Part model, mm, in its own coordinate system. Face numbers are marked on the shaded views. A direction names the side the tool comes from. Give positions to 0.01 mm unless a question says otherwise; leave off trailing zeros. Order: outer loops, then holes, each group sorted by start corner. A loop starts at its lowest first (then second) coordinate and runs counter-clockwise, first axis right, second up.
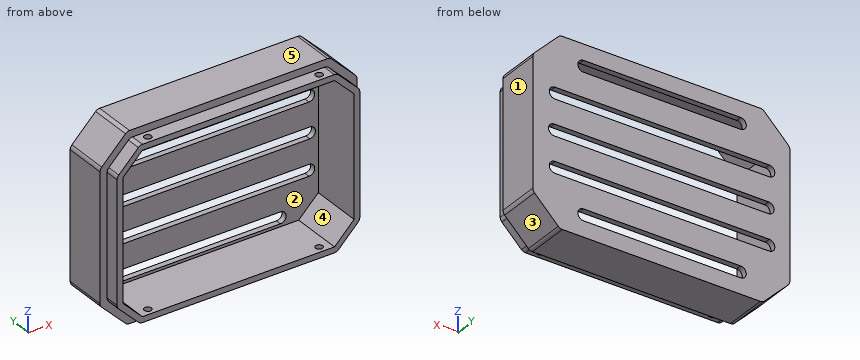
from build123d import *

# Parameters (mm, degrees)
BOSS_EXTRUDE1_DEPTH = 25.4
CUT_EXTRUDE1_DEPTH  = 6.35
CUT_EXTRUDE2_DEPTH  = 22.86
SKETCH4_R           = 1.575
CUT_EXTRUDE3_DEPTH  = 102.052823439
CUT_EXTRUDE4_DEPTH  = 75.93269063
FILLET1_R           = 2.54


with BuildPart() as part:
    # Sketch1 → Boss-Extrude1 (new body)
    with BuildSketch(Plane(origin=(0, 0, 0), x_dir=(1, 0, 0), z_dir=(0, 1, 0))):
        Polygon((-45.085, -41.275), (-57.15, -29.21), (-57.15, 29.21), (-45.085, 41.275), (45.085, 41.275), (57.15, 29.21), (57.15, -29.21), (45.085, -41.275), align=None)
    extrude(amount=BOSS_EXTRUDE1_DEPTH)

    # Sketch2 → Cut-Extrude1 (cut)
    with BuildSketch(Plane.XZ):
        Polygon((-57.15, 29.21), (-57.15, -29.21), (-45.085, -41.275), (45.085, -41.275), (57.15, -29.21), (57.15, 29.21), (45.085, 41.275), (-45.085, 41.275), align=None)
        Polygon((-53.975, 27.894871939), (-53.975, -27.894871939), (-43.769871939, -38.1), (43.769871939, -38.1), (53.975, -27.894871939), (53.975, 27.894871939), (43.769871939, 38.1), (-43.769871939, 38.1), align=None, mode=Mode.SUBTRACT)
    extrude(amount=-CUT_EXTRUDE1_DEPTH, mode=Mode.SUBTRACT)

    # Sketch3 → Cut-Extrude2 (cut)
    with BuildSketch(Plane.XZ):
        Polygon((-51.435, 26.842769491), (-51.435, -26.842769491), (-42.717769491, -35.56), (42.717769491, -35.56), (51.435, -26.842769491), (51.435, 26.842769491), (42.717769491, 35.56), (-42.717769491, 35.56), align=None)
    extrude(amount=-CUT_EXTRUDE2_DEPTH, mode=Mode.SUBTRACT)

    # Sketch4 → Cut-Extrude3 (cut, through all)
    with BuildSketch(Plane.XY.offset(38.1)):
        with Locations((-38.1, 3.175)):
            Circle(SKETCH4_R)
        with Locations((38.1, 3.175)):
            Circle(SKETCH4_R)
    extrude(amount=-CUT_EXTRUDE3_DEPTH, mode=Mode.SUBTRACT)

    # Sketch5 → Cut-Extrude4 (cut, through all)
    with BuildSketch(Plane(origin=(0, 25.4, 0), x_dir=(1, 0, 0), z_dir=(0, 1, 0))):
        with BuildLine():
            Line((-35.239850105, 34.29), (34.610149895, 34.29))
            ThreePointArc((34.610149895, 34.29), (37.150149895, 31.75), (34.610149895, 29.21))
            Line((34.610149895, 29.21), (-35.239850105, 29.21))
            ThreePointArc((-35.239850105, 29.21), (-37.779850105, 31.75), (-35.239850105, 34.29))
        make_face()
        with BuildLine():
            Line((-47.625, 2.54), (47.625, 2.54))
            ThreePointArc((47.625, 2.54), (50.165, 0), (47.625, -2.54))
            Line((47.625, -2.54), (-47.625, -2.54))
            ThreePointArc((-47.625, -2.54), (-50.165, 0), (-47.625, 2.54))
        make_face()
        with BuildLine():
            Line((-35.239850105, -29.21), (34.610149895, -29.21))
            ThreePointArc((34.610149895, -29.21), (37.150149895, -31.75), (34.610149895, -34.29))
            Line((34.610149895, -34.29), (-35.239850105, -34.29))
            ThreePointArc((-35.239850105, -34.29), (-37.779850105, -31.75), (-35.239850105, -29.21))
        make_face()
        with BuildLine():
            Line((-47.939850105, -13.335), (47.310149895, -13.335))
            ThreePointArc((47.310149895, -13.335), (49.850149895, -15.875), (47.310149895, -18.415))
            Line((47.310149895, -18.415), (-47.939850105, -18.415))
            ThreePointArc((-47.939850105, -18.415), (-50.479850105, -15.875), (-47.939850105, -13.335))
        make_face()
        with BuildLine():
            Line((-47.939850105, 18.415), (47.310149895, 18.415))
            ThreePointArc((47.310149895, 18.415), (49.850149895, 15.875), (47.310149895, 13.335))
            Line((47.310149895, 13.335), (-47.939850105, 13.335))
            ThreePointArc((-47.939850105, 13.335), (-50.479850105, 15.875), (-47.939850105, 18.415))
        make_face()
    extrude(amount=-CUT_EXTRUDE4_DEPTH, mode=Mode.SUBTRACT)

    # Fillet1
    fillet1_edges = [part.edges().sort_by_distance(p)[0] for p in [
        (-45.085, 15.875, 41.275),
        (-57.15, 15.875, 29.21),
        (-57.15, 15.875, -29.21),
        (-45.085, 15.875, -41.275),
        (45.085, 15.875, -41.275),
        (57.15, 15.875, -29.21),
        (57.15, 15.875, 29.21),
        (45.085, 15.875, 41.275),
        (-43.769871939, 3.175, 38.1),
        (43.769871939, 3.175, 38.1),
        (53.975, 3.175, 27.894871939),
        (53.975, 3.175, -27.894871939),
        (43.769871939, 3.175, -38.1),
        (-43.769871939, 3.175, -38.1),
        (-53.975, 3.175, -27.894871939),
        (-53.975, 3.175, 27.894871939),
    ]]
    fillet(fillet1_edges, radius=FILLET1_R)


solid = part.part
Item 1: Band-saw the part on A-A on x = 16. Give the number of separate pieces and of enclosed holes in the cut face, plus the area to 3 significant figures.
Item 2: Pull direction X, two halves, no side cores. Call the marked faces 3, 4 and 5: released by +X, released by -X, zero draft, split by the parting line, or undercut.
Item 3: Drill centre lines: probe 1 along X at (y, z) = (15.75, 20) (3 decimals); probe 2 along Z at (x, y) = (33.5, 23.5) (3 decimals); probe 3 along Z at (x, y) = (35, 4.25). Where is each one in solid material? Low to high.
Item 4: Band-saw the part on B-B on z = 0. List the corners of the cut face in (x, y) (3 decimals), plus the area to 3 significant figures.
Item 5: Drop flat-ended pins along their axis: P1, Ø8, axis at x = -4, z = -30.5, coming from the -Y side; P2, Ø3, axis at x = 12.5, y = 4, coming from the +Z side; P3, Ø3, axis at x = -3.5, y = 4, coming from the -Z side; P4, Ø5, axis at y = 4.5, z = 6, coming from the -X side. Give the stop position or say it passes through.
Item 6: Which spindle directions (+Z, -Z, +X, -X, +Y, -Y) get a long thin tool onto all of the face, cutting with end or side? Do the marked faces 1 and 2. Say none if no direction does.
Item 7: Band-saw the part on C-C on y = 19.75. List the corners of the cut face in (x, z) (3 decimals).
Item 8: Band-saw the part on D-D on z = 8.5. List the corners of the cut face in (x, y) (3 decimals), plus the area to 3 significant figures.
Working result:
1. separate pieces: 6
1. enclosed holes: 0
1. area: 366 mm2
2. face 3: released by +X
2. face 4: undercut
2. face 5: zero draft
3. probe 1: x = -57.15 to -51.435, 51.435 to 57.15
3. probe 2: z = -41.275 to -34.29, -29.21 to -18.415, -13.335 to -2.54, 2.54 to 13.335, 18.415 to 29.21, 34.29 to 41.275
3. probe 3: z = -38.1 to -35.56, 35.56 to 38.1
4. outline: (-57.15, 6.35) - (-53.975, 6.35) - (-53.975, 0) - (-51.435, 0) - (-51.435, 22.86) - (-50.165, 22.86) - (-50.165, 25.4) - (-57.15, 25.4) - close; (50.165, 22.86) - (51.435, 22.86) - (51.435, 0) - (53.975, 0) - (53.975, 6.35) - (57.15, 6.35) - (57.15, 25.4) - (50.165, 25.4) - close
4. area: 256 mm2
5. P1: stops at y = 22.86
5. P2: stops at z = 38.1
5. P3: stops at z = -38.1
5. P4: stops at x = -57.15
6. face 1: +Z, -Z, +X, +Y, -Y
6. face 2: -Y
7. outline: (-57.15, -28.158) arc R2.54 ccw to (-56.406, -29.954) - (-45.829, -40.531) arc R2.54 ccw to (-44.033, -41.275) - (44.033, -41.275) arc R2.54 ccw to (45.829, -40.531) - (56.406, -29.954) arc R2.54 ccw to (57.15, -28.158) - (57.15, 28.158) arc R2.54 ccw to (56.406, 29.954) - (45.829, 40.531) arc R2.54 ccw to (44.033, 41.275) - (-44.033, 41.275) arc R2.54 ccw to (-45.829, 40.531) - (-56.406, 29.954) arc R2.54 ccw to (-57.15, 28.158) - close; hole (-51.435, -26.843) - (-42.718, -35.56) - (42.718, -35.56) - (51.435, -26.843) - (51.435, 26.843) - (42.718, 35.56) - (-42.718, 35.56) - (-51.435, 26.843) - close
8. outline: (-57.15, 6.35) - (-53.975, 6.35) - (-53.975, 0) - (-51.435, 0) - (-51.435, 22.86) - (51.435, 22.86) - (51.435, 0) - (53.975, 0) - (53.975, 6.35) - (57.15, 6.35) - (57.15, 25.4) - (-57.15, 25.4) - close
8. area: 511 mm2
